The model under review builds one solid part; all positions refer to its coordinate system, in mm. Face numbers are marked on the shaded views. A direction names the side the tool comes from. Give positions to 0.01 mm unless a question says otherwise; leave off trailing zeros. Order: outer loops, then holes, each group sorted by start corner. A loop starts at its lowest first (then second) coordinate and runs counter-clockwise, first axis right, second up.
```python
from build123d import *

# Parameters (mm, degrees)
SKETCH1_R           = 66.675
BOSS_EXTRUDE1_DEPTH = 12.7
CUT_EXTRUDE1_START  = -13.7
SKETCH2_R           = 2.8575
CUT_EXTRUDE1_DEPTH  = 14.7
CIRPATTERN1_COUNT   = 8
BOSS_EXTRUDE2_DEPTH = 12.7
BOSS_EXTRUDE3_DEPTH = 6.35
CHAMFER1_SIZE       = 3.81
FILLET3_R           = 10.16
SKETCH7_R           = 10.16
BOSS_EXTRUDE4_DEPTH = 10.16
SKETCH8_R           = 19.05
BOSS_EXTRUDE5_DEPTH = 6.35
SKETCH9_R           = 6.35
BOSS_EXTRUDE6_DEPTH = 21.59
SKETCH11_W          = 2.54
SKETCH11_H          = 2.54
CUT_EXTRUDE2_DEPTH  = 2.54


with BuildPart() as part:
    # Sketch1 → Boss-Extrude1 (new body)
    with BuildSketch(Plane(origin=(0, 0, 0), x_dir=(1, 0, 0), z_dir=(0, 1, 0))):
        Circle(SKETCH1_R)
    extrude(amount=BOSS_EXTRUDE1_DEPTH)

    # Sketch2 → Cut-Extrude1 (cut)
    with BuildSketch(Plane(origin=(0, 12.7, 0), x_dir=(1, 0, 0), z_dir=(0, 1, 0)).offset(CUT_EXTRUDE1_START)):
        with Locations((0, 61.2775)):
            Circle(SKETCH2_R)
    cut_extrude1 = extrude(amount=CUT_EXTRUDE1_DEPTH, mode=Mode.SUBTRACT)

    # CirPattern1: Cut-Extrude1 ×8 about axis
    cirpattern1_axis = Axis((0, 0, 0), (0, 1, 0))
    for i in range(1, CIRPATTERN1_COUNT):
        add(cut_extrude1.rotate(cirpattern1_axis, i * 360 / CIRPATTERN1_COUNT), mode=Mode.SUBTRACT)

    # Sketch4 → Boss-Extrude2 (add)
    with BuildSketch(Plane(origin=(0, 12.7, 0), x_dir=(1, 0, 0), z_dir=(0, 1, 0))):
        Polygon((-37.08191635, 43.06228634), (-4.228760174, 56.670509195), (41.941995941, -54.795556403), (9.088839765, -68.403779258), align=None)
    extrude(amount=BOSS_EXTRUDE2_DEPTH)

    # Sketch5 → Boss-Extrude3 (add)
    with BuildSketch(Plane(origin=(0, 25.4, 0), x_dir=(1, 0, 0), z_dir=(0, 1, 0))):
        Polygon((-26.521973293, 47.436357972), (19.648782821, -64.029707626), (31.382052884, -59.169628035), (-14.78870323, 52.296437563), align=None)
    extrude(amount=BOSS_EXTRUDE3_DEPTH)

    # Chamfer1
    chamfer1_edges = [part.edges().sort_by_distance(p)[0] for p in [
        (-3.436595236, 31.75, 8.296674827),
        (8.296674827, 31.75, 3.436595236),
    ]]
    chamfer(chamfer1_edges, length=CHAMFER1_SIZE)

    # Fillet3
    fillet3_edges = [part.edges().sort_by_distance(p)[0] for p in [
        (18.856617884, 25.4, -0.937476396),
        (-13.996538293, 25.4, 12.670746459),
    ]]
    fillet(fillet3_edges, radius=FILLET3_R)

    # Sketch7 → Boss-Extrude4 (add)
    with BuildSketch(Plane(origin=(28.917473567, 0, 69.812956874), x_dir=(0.923879533, 0, -0.382683432), z_dir=(0.382683432, 0, 0.923879533))):
        with Locations((0, 15.875)):
            Circle(SKETCH7_R)
    extrude(amount=-BOSS_EXTRUDE4_DEPTH)

    # Sketch8 → Boss-Extrude5 (add)
    with BuildSketch(Plane(origin=(28.917473567, 0, 69.812956874), x_dir=(0.923879533, 0, -0.382683432), z_dir=(0.382683432, 0, 0.923879533))):
        with Locations((0, 15.875)):
            Circle(SKETCH8_R)
    extrude(amount=BOSS_EXTRUDE5_DEPTH)

    # Sketch9 → Boss-Extrude6 (add)
    with BuildSketch(Plane(origin=(31.347513362, 0, 75.679591906), x_dir=(0.923879533, 0, -0.382683432), z_dir=(0.382683432, 0, 0.923879533))):
        with Locations((0, 15.875)):
            Circle(SKETCH9_R)
    extrude(amount=BOSS_EXTRUDE6_DEPTH)

    # Sketch11 → Cut-Extrude2 (cut)
    with BuildSketch(Plane(origin=(39.609648667, 0, 95.626151013), x_dir=(0.923879533, 0, -0.382683432), z_dir=(0.382683432, 0, 0.923879533))):
        with Locations((0, 15.875)):
            Rectangle(SKETCH11_W, SKETCH11_H)
    extrude(amount=-CUT_EXTRUDE2_DEPTH, mode=Mode.SUBTRACT)


solid = part.part
```
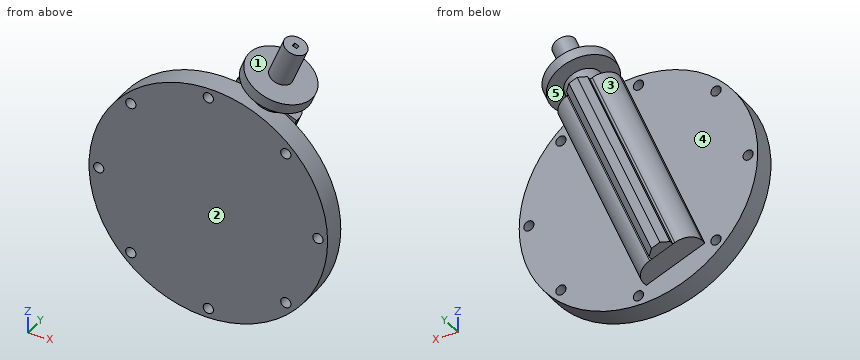
1. Take a section at A-A (y = 19). Write out the cut boundary in (x, z) (3 decimals).
2. Take a section at B-B (x = 0). Count the separate pieces of the cut face and the enclosed holes in it, and give its area (3 significant figures).
3. To check wall thickness, follow line 1 (X direction, y = 11, z = 0.5); line 2 (X direction, y = 9, z = 0) (3 decimals); line 3 (Y direction, x = -8.5, z = 57). State the ranges of each line that lie inside material, in increasing order.
4. For the marked faces 4 and 5, list the 3-axis set-ups (+Z, -Z, +X, -X, +Y, -Y) from which the entire face can be reached by the end or side of a thin tool; tool diameter is ignored.
5. Take a section at D-D (x = -55). Write out the cut boundary in (y, z), and give its area (3 significant figures).
6. Draft analysis for pull direction X (two halves, no side actions). For the marked faces 1, 2 and 3, state which applies: pulls with the +X half, pulls with the -X half, needs draft (parallel to the pull), parting line crosses it, or undercut.
7. Insertion check: pin 1 (6 mm diameter, centred on y = 8, z = 47, fed in from -X); pin 2 (8 mm diameter, centred on x = 6.5, z = -23.5, fed in from -Y); pin 3 (7.5 mm diameter, centred on x = 0, z = -61.28, fed in from +Y); pin 4 (4.5 mm diameter, centred on x = 61.28, z = 0, fed in from -Y). Each pin has a flat end and moves straight along its axis. Give the tip position at first contact, or say it passes through.
Answer:
1. outline: (-36.415, -43.338) - (-4.895, -56.394) - (41.276, 55.072) - (34.447, 57.9) - (37.849, 66.113) - (46.279, 62.622) - (48.709, 68.488) - (36.455, 73.564) - (44.717, 93.511) - (34.503, 97.742) - (26.24, 77.795) - (13.986, 82.871) - (11.556, 77.004) - (19.986, 73.513) - (16.584, 65.299) - (9.755, 68.128) - close
2. separate pieces: 3
2. enclosed holes: 0
2. area: 2,790 mm2
3. line 1: x = -66.67 to -64.09, -58.46 to 58.46, 64.09 to 66.67
3. line 2: x = -66.675 to -64.135, -58.42 to 58.42, 64.135 to 66.675
3. line 3: y = 0 to 12.7
4. face 4: +Y
4. face 5: none
5. outline: (0, -37.69) - (12.7, -37.69) - (12.7, 37.69) - (0, 37.69) - close
5. area: 957 mm2
6. face 1: undercut
6. face 2: needs draft
6. face 3: pulls with the -X half
7. pin 1: stops at x = -50.1
7. pin 2: stops at y = 0
7. pin 3: stops at y = 12.7
7. pin 4: passes through
